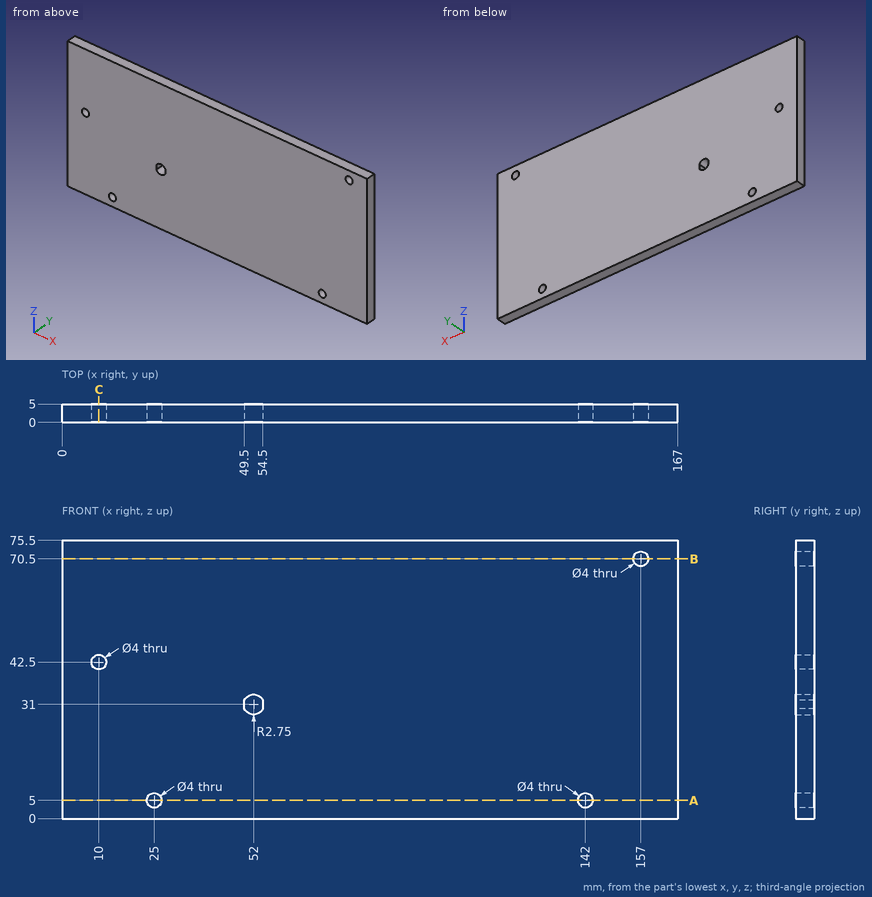
Verification items for this drawing (mm, ordinates from the low corner). Coordinates: 2 decimals unless noted, no trailing zeros. Loops run counter-clockwise (first coordinate to the right, second up) from the corner with the lowest first, then second, coordinate; pieces in that order, holes last. Notation, with made-up numbers: (67.25, 30.5) - (116.25, 30.5) arc R22 cw to (116.25, 47.5) - close; hole circle Ø1 at (-17.75, 74.5). An arc over 180 degrees is marked (long way). Use one line per item in the form item = value. Start each with the question number.
Item 1: Section check A-A, the plane z = 5. Enter the section's corners in (x, y).
Item 2: Thickness scan on probe 1 along X at (y, z) = (1.3, 5); probe 2 along Z at (x, y) = (142, 2.3); probe 3 along X at (y, z) = (3.15, 42.5). Record the ranges inside material, lowest first.
Item 3: Section check B-B, the plane z = 70.5. Enter the section's corners in (x, y), and give its area (3 significant figures).
Item 4: Gauge pin test, flat end, axial feed: pin 1 (3.5 mm diameter, centred on x = 25, z = 5, fed in from -Y). Record the tip position at first contact, or that the pin passes through.
Item 5: Section check C-C, the plane x = 10. Enter the section's corners in (y, z).
Computed:
q1.outline = (0, 0) - (23, 0) - (23, 5) - (0, 5) - close; (27, 0) - (140, 0) - (140, 5) - (27, 5) - close; (144, 0) - (167, 0) - (167, 5) - (144, 5) - close
q2.probe_1 = 0 to 23, 27 to 140, 144 to 167
q2.probe_2 = 0 to 3, 7 to 75.5
q2.probe_3 = 0 to 8, 12 to 167
q3.outline = (0, 0) - (155, 0) - (155, 5) - (0, 5) - close; (159, 0) - (167, 0) - (167, 5) - (159, 5) - close
q3.area = 815 mm2
q4.pin_1 = through
q5.outline = (0, 0) - (5, 0) - (5, 40.5) - (0, 40.5) - close; (0, 44.5) - (5, 44.5) - (5, 75.5) - (0, 75.5) - close
